from build123d import *

# Parameters (mm, degrees)
EXTRUDE_1_DEPTH        = 120
SKETCH_3_W             = 120
SKETCH_3_H             = 20
SM_BASE_FLANGE_1_DEPTH = 3
SM_EDGE_FLANGE_1_DEPTH = 20
EXTRUDE_1_2_DEPTH      = 3


# Sheet-metal steps are written as plain solids
with BuildPart() as part:
    # Sketch 1 → Extrude 1 (new body)
    with BuildSketch(Plane(origin=(0, 0, 0), x_dir=(0, 0, -1), z_dir=(1, 0, 0))):
        Polygon((0, 20), (0, 0), (20, 0), (20, 3), (3, 3), (3, 20), align=None)
    extrude(amount=EXTRUDE_1_DEPTH)



with BuildPart() as body_2:
    # Эскиз3 → Базовая кромка1 (new body)
    with BuildSketch(Plane.XZ):
        with Locations((60, -10)):
            Rectangle(SKETCH_3_W, SKETCH_3_H)
    extrude(amount=-SM_BASE_FLANGE_1_DEPTH)

    # Ребро-кромка1 section (across the edge) → Ребро-кромка1 (add)
    with BuildSketch(Plane(origin=(-0.520567051, 0, 0), x_dir=(0.8191520442889892, -0.5735764363510499, 0), z_dir=(0, 0, -1))):
        with BuildLine():
            Line((-3, 0.520567051), (-3, 23.438298848))
            Line((-3, 23.438298848), (0, 23.438298848))
            Line((0, 23.438298848), (0, 0.520567051))
            ThreePointArc((0, 0.520567051), (0.112989167, 0.058818437), (0.426423564, -0.298584994))
            Line((0.426423564, -0.298584994), (-1.294305745, -2.756041127))
            ThreePointArc((-1.294305745, -2.756041127), (-2.548043333, -1.326427402), (-3, 0.520567051))
        make_face()
    extrude(amount=SM_EDGE_FLANGE_1_DEPTH)


with BuildPart() as part_1:
    add(part.part)

    add(body_2.part)  # Extrude 1 2 merges body 2
    # Эскиз11 → Extrude 1 2 (add)
    with BuildSketch(Plane.XY):
        Polygon((0, 20), (0, 3), (-12.829726495, 11.983471205), (-7.216492602, 20), align=None)
    extrude(amount=-EXTRUDE_1_2_DEPTH)


solid = part_1.part
Could you check a few things on this model? Use its own coordinates, in mm. A direction names the side the tool comes from. Coordinates: 2 decimals unless noted, no trailing zeros. Order: outer loops, then holes, each group sorted by start corner. A loop starts at its lowest first (then second) coordinate and runs counter-clockwise, first axis right, second up. Notation, with made-up numbers: (-26, -26) -> (-10, -26) arc R4 ccw to (-10, -22) -> close; hole circle Ø11 at (75, 61). An arc over 180 degrees is marked (long way). One line per item, written item: value. Start each with the question number.
1) Imagine slicing it at B-B on x = 106.5. List the corners of the cut face in (y, z) for me.
2) Imagine slicing it at A-A on z = -1.75. List the corners of the cut face in (x, y) for me.
3) Imagine slicing it at D-D on y = 5.5. List the corners of the cut face in (x, z) for me, plus the area to 3 significant figures.
4) If I drill on L1, parallel to Y at x = 26.5, z = -12.25; L2, parallel to Z at x = 91, y = 9; L3, parallel to X at y = 1, z = -7.25, over which ranges is the centre line in solid material (lowest first)? Write a range as [from, to].
5) Which directions (+Z, -Z, +X, -X, +Y, -Y) give clear straight access to the entire face, cutting with the end or side of a thin tool? Please do faces 4 (the flat face through (59, 0, -10)), 5 (the flat face through (59, 3, -12)), 6 (the flat face through (56, 20, -1)).
6) We'd pull the mould along Y, two halves only. Please class faces 1 (the flat face through (-7.48, -9.94, -9.86)), 2 (the flat face through (-6.33, 7.43, -1.48)), 3 (the flat face through (55, 12, -3)): +Y half, -Y half, draft (parallel to the pull), parting line (faces both ways), or undercut.
7) I'm going to push flat-ended pins straight in: pin 1 (8 mm diameter, centred on y = 1.5, z = -6.5, fed in from -X); pin 2 (12 mm diameter, centred on y = -4, z = -7.5, fed in from -X); pin 3 (13.5 mm diameter, centred on x = 48, y = 10, fed in from -Z). Where does each tip first touch, or does it pass through?
8) Imagine slicing it at C-C on z = -14.75. List the corners of the cut face in (x, y) for me, plus the area to 3 significant figures.
Answer list:
1. outline: (0, -20) -> (3, -20) -> (3, -3) -> (20, -3) -> (20, 0) -> (0, 0) -> close
2. outline: (-16.42, -17.48) -> (-13.96, -19.2) -> (-0.82, -0.43) arc R1 cw to (0, 0) -> (120, 0) -> (120, 20) -> (-7.22, 20) -> (-12.83, 11.98) -> (0, 3) arc R4 ccw to (-3.28, 1.29) -> close
3. outline: (-3.57, -3) -> (120, -3) -> (120, 0) -> (-3.57, 0) -> close
3. area: 371 mm2
4. L1: y = [0, 3]
4. L2: z = [-3, 0]
4. L3: x = [-3.48, 120]
5. face 4: +Z, -Z, +X, -Y
5. face 5: -Z, +X, -X, +Y
5. face 6: +Z, -Z, +X, -X, +Y
6. face 1: -Y half
6. face 2: undercut
6. face 3: draft
7. pin 1: stops at x = -5.93
7. pin 2: stops at x = -11.18
7. pin 3: stops at z = -3
8. outline: (-16.42, -17.48) -> (-13.96, -19.2) -> (-0.82, -0.43) arc R1 cw to (0, 0) -> (120, 0) -> (120, 3) -> (0, 3) arc R4 ccw to (-3.28, 1.29) -> close
8. area: 436 mm2
